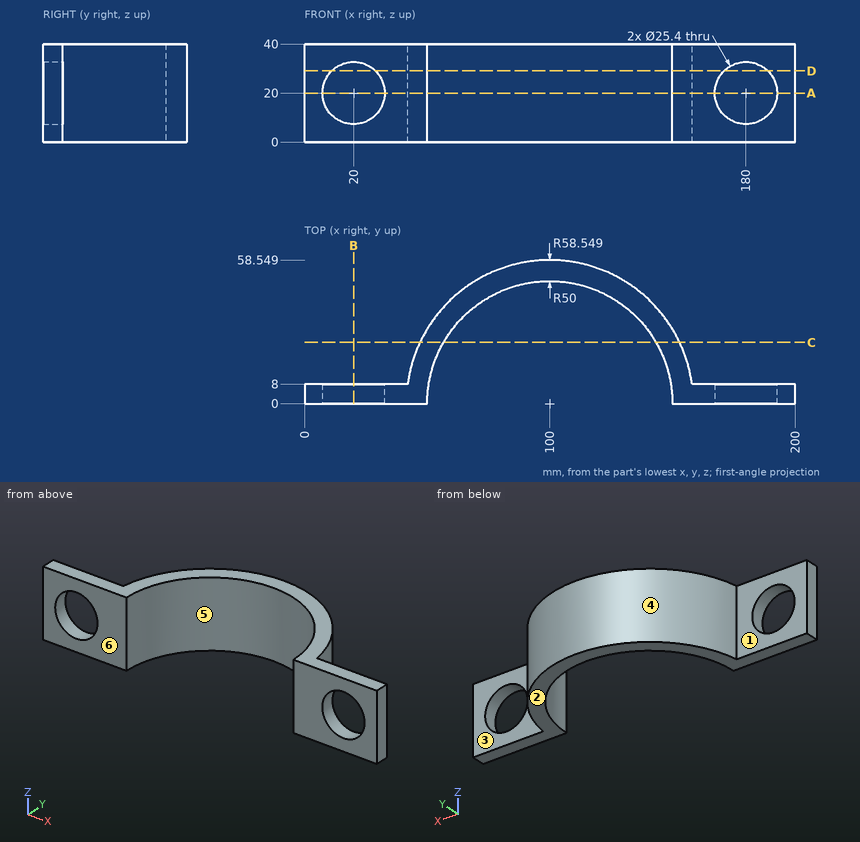
Here's the drawing with two shaded views (mm, measured from the low corner). I have some questions. A direction names the side the tool comes from. Round coordinates to 2 decimals unless told otherwise and drop trailing zeros. Order: outer loops, then holes, each group sorted by start corner. A loop starts at its lowest first (then second) coordinate and runs counter-clockwise, first axis right, second up. Notation, with made-up numbers: (-29.5, 30) -> (7.5, 30) arc R27 cw to (7.5, 69) -> close; hole circle Ø4 at (16, 20). An arc over 180 degrees is marked (long way). Use a Markdown table: item, result. Add a question column.
(1) Suppose I cut it at A-A, the plane z = 20. Please give me the cut outline in (x, y), and give its area (3 significant figures).
(2) For pin 1 Ø10 at (x, z) = (125.5, 32) entering from -Y; pin 2 Ø10 at (x, y) = (63.5, 49.5) entering from -Z; pin 3 Ø4 at (x, z) = (128, 5.5) entering from -Y; pin 4 Ø10 at (y, z) = (23, 26.5) entering from -X, each with a flat end and sliding along its axis, tell me the tip position at first contact or that it passes through.
(3) Suppose I cut it at B-B, the plane x = 20. Please give me the cut outline in (y, z).
(4) I need wall thicknesses on line 1 along Z through (x, y) = (20, 6); line 2 along X through (y, z) = (31.5, 32); line 3 along X through (y, z) = (8.5, 12). Which ranges of each line are inside material? Lowest first, please.
(5) Suppose I cut it at C-C, the plane y = 25. Please give me the cut outline in (x, z), and give its area (3 significant figures).
(6) If we mould it in two halves opening along X, with no side actions, what happens to the marked faces 4, 5 and 6? For each: released by +X, released by -X, zero draft, split by the parting line, or undercut.
(7) Suppose I cut it at D-D, the plane z = 29. Please give me the cut outline in (x, y).
(8) For the marked faces 1, 2 and 3, which set-ups out of +Z, -Z, +X, -X, +Y, -Y let a thin tool reach every point of the face, with its end or its side?
Verdict:
| question | item | result |
|---|---|---|
| 1 | outline | (0, 0) -> (7.3, 0) -> (7.3, 8) -> (0, 8) -> close; (32.7, 0) -> (50, 0) arc R50 cw to (150, 0) -> (167.3, 0) -> (167.3, 8) -> (158, 8) arc R58.55 ccw to (42, 8) -> (32.7, 8) -> close; (192.7, 0) -> (200, 0) -> (200, 8) -> (192.7, 8) -> close |
| 1 | area | 1,720 mm2 |
| 2 | pin 1 | y = 39.62 |
| 2 | pin 2 | z = 0 |
| 2 | pin 3 | y = 40 |
| 2 | pin 4 | x = 44.29 |
| 3 | outline | (0, 0) -> (8, 0) -> (8, 7.3) -> (0, 7.3) -> close; (0, 32.7) -> (8, 32.7) -> (8, 40) -> (0, 40) -> close |
| 4 | line 1 | 0 to 7.3, 32.7 to 40 |
| 4 | line 2 | 50.65 to 61.17, 138.83 to 149.35 |
| 4 | line 3 | 42.07 to 50.73, 149.27 to 157.93 |
| 5 | outline | (47.06, 0) -> (56.7, 0) -> (56.7, 40) -> (47.06, 40) -> close; (143.3, 0) -> (152.94, 0) -> (152.94, 40) -> (143.3, 40) -> close |
| 5 | area | 771 mm2 |
| 6 | face 4 | split by the parting line |
| 6 | face 5 | undercut |
| 6 | face 6 | zero draft |
| 7 | outline | (0, 0) -> (11.04, 0) -> (11.04, 8) -> (0, 8) -> close; (28.96, 0) -> (50, 0) arc R50 cw to (150, 0) -> (171.04, 0) -> (171.04, 8) -> (158, 8) arc R58.55 ccw to (42, 8) -> (28.96, 8) -> close; (188.96, 0) -> (200, 0) -> (200, 8) -> (188.96, 8) -> close |
| 8 | face 1 | +Z, -Z, -X, +Y |
| 8 | face 2 | -Z, +X, -X, +Y, -Y |
| 8 | face 3 | +Z, -Z, +X, +Y |
